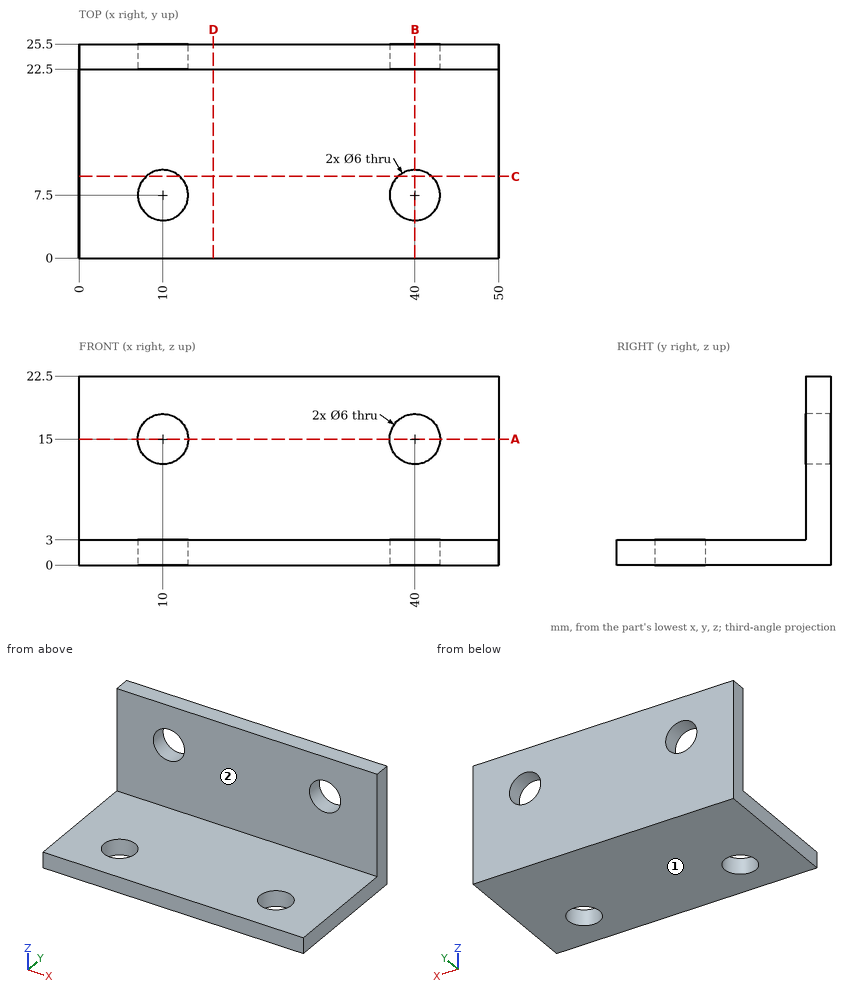
Could you check a few things on this drawing? It's one solid part, dimensions in mm from its lowest x, y, z. A direction names the side the tool comes from. Round coordinates to 2 decimals unless told otherwise and drop trailing zeros. Write each loop counter-clockwise with the first axis right and the second up, starting at its lowest first coordinate (ties: lowest second). Pieces come first, ordered by that corner, then holes. Notation, with made-up numbers: (47.25, -6.75) -> (56.25, -6.75) arc R26 cw to (56.25, 27.25) -> close; hole circle Ø2 at (25, -15). An arc over 180 degrees is marked (long way). Use one line per item in the form item = value. Start each with the question number.
Q1. Imagine slicing it at D-D (x = 16). Please give me the cut outline in (y, z).
Q2. I'm going to push flat-ended pins straight in: P1, Ø9.5, axis at x = 10, y = 7.5, coming from the +Z side; P2, Ø3, axis at x = 38, z = 19, coming from the -Y side. Where does each tip first touch, or does it pass through?
Q3. Imagine slicing it at A-A (z = 15). Please give me the cut outline in (x, y), then the cut area to 3 significant figures.
Q4. Which directions (+Z, -Z, +X, -X, +Y, -Y) give clear straight access to the entire face, cutting with the end or side of a thin tool? Please do the marked faces 1 and 2.
Q5. If I drill on probe 1 along X at (y, z) = (24.3, 15); probe 2 along Z at (x, y) = (10, 23.3); probe 3 along X at (y, z) = (24, 13), over which ranges is the centre line in solid material (lowest first)? Write a range as [from, to].
Q6. Imagine slicing it at C-C (y = 9.75). Please give me the cut outline in (x, z).
Q7. Imagine slicing it at B-B (x = 40). Please give me the cut outline in (y, z), then the cut area to 3 significant figures.
Worked out:
q1.outline = (0, 0) -> (25.5, 0) -> (25.5, 22.5) -> (22.5, 22.5) -> (22.5, 3) -> (0, 3) -> close
q2.P1 = 3
q2.P2 = 22.5
q3.outline = (0, 22.5) -> (7, 22.5) -> (7, 25.5) -> (0, 25.5) -> close; (13, 22.5) -> (37, 22.5) -> (37, 25.5) -> (13, 25.5) -> close; (43, 22.5) -> (50, 22.5) -> (50, 25.5) -> (43, 25.5) -> close
q3.area = 114 mm^2
q4.face_1 = -Z, +X, -X, +Y, -Y
q4.face_2 = +Z, +X, -X, -Y
q5.probe_1 = [0, 7], [13, 37], [43, 50]
q5.probe_2 = [0, 12], [18, 22.5]
q5.probe_3 = [0, 7.76], [12.24, 37.76], [42.24, 50]
q6.outline = (0, 0) -> (8.02, 0) -> (8.02, 3) -> (0, 3) -> close; (11.98, 0) -> (38.02, 0) -> (38.02, 3) -> (11.98, 3) -> close; (41.98, 0) -> (50, 0) -> (50, 3) -> (41.98, 3) -> close
q7.outline = (0, 0) -> (4.5, 0) -> (4.5, 3) -> (0, 3) -> close; (10.5, 0) -> (25.5, 0) -> (25.5, 12) -> (22.5, 12) -> (22.5, 3) -> (10.5, 3) -> close; (22.5, 18) -> (25.5, 18) -> (25.5, 22.5) -> (22.5, 22.5) -> close
q7.area = 99.0 mm^2
